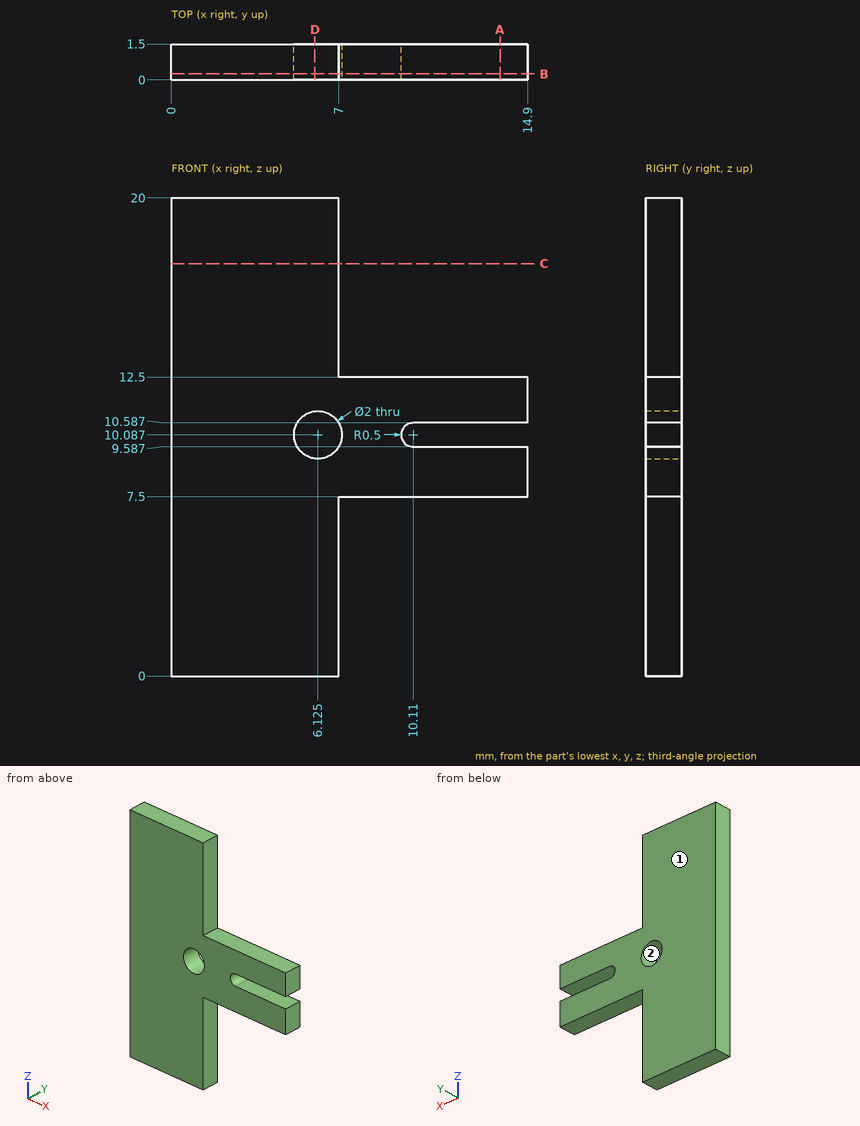
Job drawing, mm, ordinate dimensions from the low corner. One solid piece. Coordinates: 2 decimals unless noted, no trailing zeros. Write each loop counter-clockwise with the first axis right and the second up, starting at its lowest first coordinate (ties: lowest second). Pieces come first, ordered by that corner, then holes.
Item 1: Slice it at C-C (z = 17.25). Write the cut outline in (x, y), and give its area (3 significant figures).
Item 2: Mould opens along X. For the marked faces 1 and 2 say: released by +X, released by -X, zero draft, split by the parting line, or undercut.
Item 3: Slice it at B-B (y = 0.25). Write the cut outline in (x, z) (1 decimal), and give its area (3 significant figures).
Item 4: Pin check, flat tips, straight feed: pin 1 (0.8 mm diameter, centred on x = 13, y = 1, fed in from -Z); pin 2 (8 mm diameter, centred on x = 3, z = 5.5, fed in from -Y); pin 3 (1.8 mm diameter, centred on x = 6.13, z = 10.09, fed in from +Y); pin 4 (0.8 mm diameter, centred on y = 1, z = 15.5, fed in from +X). Stop position of each tip, or through.
Item 5: Slice it at D-D (x = 6). Write the cut outline in (y, z) (1 decimal).
Item 6: Probe line 1 (Z direction, x = 12.25, y = 0.4); line 2 (X direction, y = 1.25, z = 14); line 3 (Z direction, x = 5.5, y = 0.2) (1 decimal). List the from-to ranges inside material, lowest first.
Item 7: Slice it at A-A (x = 13.75). Write the cut outline in (y, z).
Results found:
1. outline: (0, 0) - (7, 0) - (7, 1.5) - (0, 1.5) - close
1. area: 10.5 mm2
2. face 1: zero draft
2. face 2: undercut
3. outline: (0, 0) - (7, 0) - (7, 7.5) - (14.9, 7.5) - (14.9, 9.6) - (10.1, 9.6) arc R0.5 cw to (10.1, 10.6) - (14.9, 10.6) - (14.9, 12.5) - (7, 12.5) - (7, 20) - (0, 20) - close; hole circle Ø2 at (6.1, 10.1)
3. area: 171 mm2
4. pin 1: stops at z = 7.5
4. pin 2: stops at y = 0
4. pin 3: passes through
4. pin 4: stops at x = 7
5. outline: (0, 0) - (1.5, 0) - (1.5, 9.1) - (0, 9.1) - close; (0, 11.1) - (1.5, 11.1) - (1.5, 20) - (0, 20) - close
6. line 1: z = 7.5 to 9.59, 10.59 to 12.5
6. line 2: x = 0 to 7
6. line 3: z = 0 to 9.3, 10.9 to 20
7. outline: (0, 7.5) - (1.5, 7.5) - (1.5, 9.59) - (0, 9.59) - close; (0, 10.59) - (1.5, 10.59) - (1.5, 12.5) - (0, 12.5) - close
